from build123d import *

# Parameters (mm, degrees)
Y_KSEKLIK_EKSTR_ZYON1_DEPTH = 3
IZIM2_R                     = 1.5
KES_EKSTR_ZYON1_DEPTH       = 12.5


with BuildPart() as part:
    # Çizim1 → Yükseklik-Ekstrüzyon1 (new body)
    with BuildSketch(Plane.XY):
        with BuildLine():
            Line((-50, 7.5), (-33.453317398, 7.5))
            ThreePointArc((-33.453317398, 7.5), (-18.650063238, -0.147459849), (-2.048249465, -1.561586909))
            ThreePointArc((-2.048249465, -1.561586909), (13.901303084, 0.11670329), (28.138290623, 7.5))
            ThreePointArc((28.138290623, 7.5), (29.856514488, 3.351840642), (28.138290623, -0.796318716))
            ThreePointArc((28.138290623, -0.796318716), (14.826618758, -5.799776605), (0.707679736, -7.5))
            Line((0.707679736, -7.5), (-50, -7.5))
            ThreePointArc((-50, -7.5), (-57.5, 0), (-50, 7.5))
        make_face()
    extrude(amount=Y_KSEKLIK_EKSTR_ZYON1_DEPTH)

    # Çizim2 → Kes-Ekstrüzyon1 (cut)
    with BuildSketch(Plane.XY.offset(3)):
        with Locations((-50, 0)):
            Circle(IZIM2_R)
    extrude(amount=-KES_EKSTR_ZYON1_DEPTH, mode=Mode.SUBTRACT)


solid = part.part
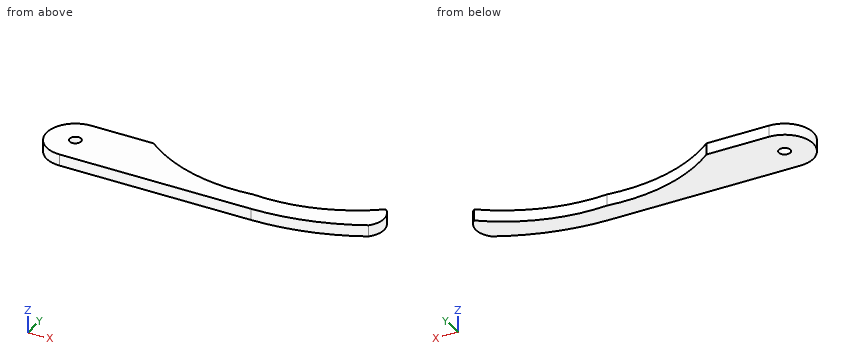
Verification items for the finished model (mm, model axes). Coordinates: 2 decimals unless noted, no trailing zeros. Order: outer loops, then holes, each group sorted by start corner. A loop starts at its lowest first (then second) coordinate and runs counter-clockwise, first axis right, second up. Notation, with made-up numbers: M 40,-11.75 L 80,-11.75 A16 ccw 80,13.25 Z; hole C -14.5,21.5 d10. An arc over 180 degrees is marked long. One line per item, written item: value. Start each with the question number.
Item 1: Sectioned sample at B-B on z = 0.65. Record the cut outline in (x, y).
Item 2: Thickness scan on probe 1 along Y at (x, z) = (-50, 0.75); probe 2 along X at (y, z) = (2, 2); probe 3 along X at (y, z) = (6.25, 0.2). Record the ranges inside material, lowest first.
Item 3: Sectioned sample at D-D on x = 4. Record the cut outline in (y, z).
Item 4: Sectioned sample at A-A on y = 6.75. Record the cut outline in (x, z), then the cut area to 3 significant figures.
Item 5: Sectioned sample at C-C on y = 0. Record the cut outline in (x, z).
Calculated:
1. outline: M -50,-7.5 L 0.71,-7.5 A59.47 ccw 28.14,-0.8 A5.87 ccw 28.14,7.5 A43.18 cw -2.05,-1.56 A42.79 cw -33.45,7.5 L -50,7.5 A7.5 ccw Z; hole C -50,0 d3
2. probe 1: -7.5 to -1.5, 1.5 to 7.5
2. probe 2: -57.23 to -24.47, 18.99 to 29.7
2. probe 3: -54.15 to -31.8, 26.46 to 29.09
3. outline: M -7.41,0 L -1.63,0 L -1.63,3 L -7.41,3 Z
4. outline: M -53.27,0 L -32.48,0 L -32.48,3 L -53.27,3 Z; M 27.15,0 L 28.77,0 L 28.77,3 L 27.15,3 Z
4. area: 67.2 mm^2
5. outline: M -57.5,0 L -51.5,0 L -51.5,3 L -57.5,3 Z; M -48.5,0 L -19.15,0 L -19.15,3 L -48.5,3 Z; M 13.51,0 L 28.8,0 L 28.8,3 L 13.51,3 Z
